CAD build for the part. Positions are in the model's coordinates, mm. Give positions to 0.01 mm unless a question says otherwise; leave off trailing zeros. Order: outer loops, then holes, each group sorted by start corner. A loop starts at its lowest first (then second) coordinate and runs counter-clockwise, first axis right, second up. Notation, with made-up numbers: M 37,-34.5 L 96,-34.5 A5 cw 96,-28.5 Z; hole C 60.5,-24.5 d4. An arc over 180 degrees is marked long. Put each result on its own line as item: value. Start each with the question number.
1) Cut at A-A (z = 261.5). Write the cut outline in (x, y) (3 decimals), and give its area (3 significant figures).
2) Drill centre lines: line 1 (Y direction, x = 0.5, z = 215.9) (3 decimals); line 2 (X direction, y = 5, z = 55.5). Where is each one in solid material? Low to high. Write a range as [from, to].
3) Cut at B-B (x = 4). Write the cut outline in (y, z).
4) Pin check, flat tips, straight feed: pin 1 (1 mm diameter, centred on x = 2, z = 83.5, fed in from +Y); pin 2 (2.5 mm diameter, centred on y = 8.33, z = 422.28, fed in from -X); pin 3 (7.5 mm diameter, centred on y = 7, z = 306, fed in from +X). Stop position of each tip, or through.
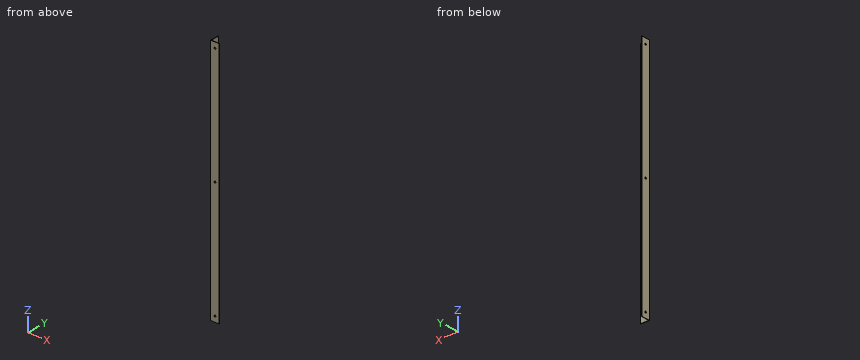
Autodesk Inventor part; units mm, degrees
ref_plane "YZ Plane" through (0, 0, 0) normal (1, 0, 0) x (0, 1, 0)
ref_plane "XZ Plane" through (0, 0, 0) normal (0, 1, 0) x (-1, 0, 0)
ref_plane "XY Plane" through (0, 0, 0) normal (0, 0, 1) x (1, 0, 0)
sketch "Sketch1" plane through (0, 0, 0) normal (0, 0, 1) x (1, 0, 0)
  line L0 (0, 0) -> (0, 15.875)
  line L1 (0, 15.875) -> (0.7937, 15.875)
  line L2 (0.7937, 15.875) -> (0.7938, 0.7937)
  line L3 (0.7938, 0.7937) -> (15.875, 0.7937)
  line L4 (15.875, 0.7937) -> (15.875, 0)
  line L5 (15.875, 0) -> (0, 0)
  dimension "d0" = 15.875
  dimension "d1" = 0.7937
extrude "Extrusion1" add sketch "Sketch1" along normal blind 431.8
sketch "Sketch2" plane through (0.7938, 0.7937, 0) normal (0, 1, 0) x (1, 0, 0)
  line L0 (0, 0) -> (15.0812, 0)
  line L1 (15.0812, -431.8) -> (0, -431.8)
  line L2 (7.5406, 0) -> (7.5406, -431.8) construction
  circle A0 centre (7.5406, -9.525) radius 1.5875
  circle A1 centre (7.5406, -215.9) radius 1.5875
  circle A2 centre (7.5406, -422.275) radius 1.5875
  point P0 (-0.7938, 0)
  dimension "d4" = 9.525
  dimension "d5" = 3.175
  dimension "d6" = 431.8
  dimension "d9" = 206.375
sketch "Sketch3" plane through (0.7938, 0.7937, 0) normal (1, 0, 0) x (0, 0, -1)
  line L0 (0, 15.0812) -> (0, 0)
  line L1 (-431.8, 0) -> (-431.8, 15.0812)
  line L2 (-431.8, 7.5406) -> (0, 7.5406) construction
  circle A0 centre (-9.525, 7.5406) radius 1.5875
  circle A1 centre (-215.9, 7.5406) radius 1.5875
  circle A2 centre (-422.275, 7.5406) radius 1.5875
  point P0 (0, -0.7937)
  dimension "d14" = 3.175
  dimension "d15" = 9.525
  dimension "d16" = 431.8
  dimension "d19" = 206.375
extrude "Extrusion2" cut sketch "Sketch2" against normal through all
extrude "Extrusion3" cut sketch "Sketch3" against normal through all
properties part number "Hopper Bracing Front Top P8" material "Aluminum 6061"
Solution:
1. outline: M 0,0 L 15.875,0 L 15.875,0.794 L 0.794,0.794 L 0.794,15.875 L 0,15.875 Z
1. area: 24.6 mm²
2. line 1: [0, 6.747], [9.922, 15.875]
2. line 2: [0, 0.79]
3. outline: M 0,0 L 0.79,0 L 0.79,431.8 L 0,431.8 Z
4. pin 1: y = 0.79
4. pin 2: through
4. pin 3: x = 0.79
